```python
from build123d import *

# Parameters (mm, degrees)
SKETCH1_R           = 6.2
BOSS_EXTRUDE1_DEPTH = 5.4
SKETCH2_R           = 3
BOSS_EXTRUDE3_DEPTH = 102.1
BOSS_EXTRUDE4_START = 5.4
SKETCH4_R           = 6.2
BOSS_EXTRUDE4_DEPTH = 5.4
SKETCH5_R           = 6
BOSS_EXTRUDE5_DEPTH = 43.8


with BuildPart() as part:
    # Sketch1 → Boss-Extrude1 (new body)
    with BuildSketch(Plane.XY):
        with BuildLine():
            Line((0, 0), (-149.578947368, 0))
            ThreePointArc((-149.578947368, 0), (-174.878947368, -25.3), (-149.578947368, -50.6))
            Line((-149.578947368, -50.6), (130.421052632, -50.6))
            ThreePointArc((130.421052632, -50.6), (155.721052632, -25.3), (130.421052632, 0))
            Line((130.421052632, 0), (0, 0))
        make_face()
        with Locations(Location((130.421052632, -25.3, 0), (0, 0, 180))):
            Circle(SKETCH1_R, mode=Mode.SUBTRACT)
    extrude(amount=BOSS_EXTRUDE1_DEPTH)

    # Sketch2 → Boss-Extrude3 (add)
    with BuildSketch(Plane(origin=(0, 0, 0), x_dir=(-1, 0, 0), z_dir=(0, 0, -1))):
        with Locations(Location((-68.985809966, -25.3, 0), (0, 0, 180))):
            Circle(SKETCH2_R)
    extrude(amount=BOSS_EXTRUDE3_DEPTH)

    # Sketch4 → Boss-Extrude4 (add)
    with BuildSketch(Plane(origin=(0, 0, -102.1), x_dir=(-1, 0, 0), z_dir=(0, 0, -1)).offset(BOSS_EXTRUDE4_START)):
        with BuildLine():
            Line((-130.421052632, 0), (149.578947368, 0))
            ThreePointArc((149.578947368, 0), (174.878947368, -25.3), (149.578947368, -50.6))
            Line((149.578947368, -50.6), (-130.421052632, -50.6))
            ThreePointArc((-130.421052632, -50.6), (-155.721052632, -25.3), (-130.421052632, 0))
        make_face()
        with Locations((-130.421052632, -25.3)):
            Circle(SKETCH4_R, mode=Mode.SUBTRACT)
    extrude(amount=-BOSS_EXTRUDE4_DEPTH)

    # Sketch5 → Boss-Extrude5 (add)
    with BuildSketch(Plane.XY.offset(-102.1)):
        with Locations((-149.578947368, -25.3)):
            Circle(SKETCH5_R)
    boss_extrude5 = extrude(amount=BOSS_EXTRUDE5_DEPTH)

    # Mirror1: Boss-Extrude5 across plane
    add(boss_extrude5.mirror(Plane.XY.offset(-51.05)))


solid = part.part
```
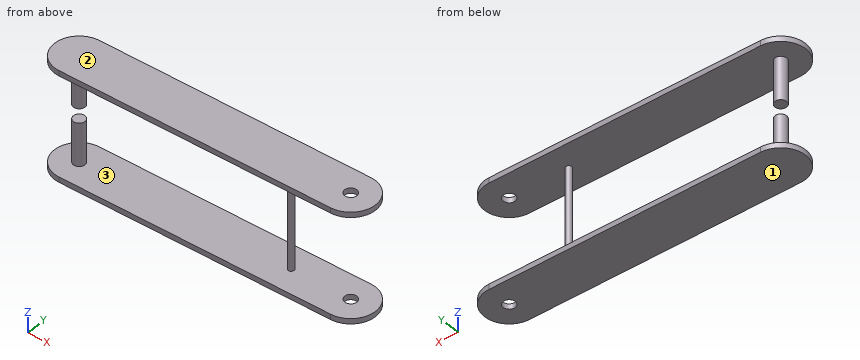
Source: CAD feature listing. Evaluate the final solid. Frame: model axes, mm. Face numbers are marked on the shaded views. Round coordinates to 2 decimals unless told otherwise and drop trailing zeros. Write each loop counter-clockwise with the first axis right and the second up, starting at its lowest first coordinate (ties: lowest second). Pieces come first, ordered by that corner, then holes. Notation, with made-up numbers: M 65.5,-20.75 L 94.5,-20.75 A26 ccw 94.5,8.25 Z; hole C 73.5,-19.75 d8. An arc over 180 degrees is marked long. Use CSV: the item, a comma, the result in double quotes. Start each with the question number.
Q1. Pull-direction query (Z, two-part tool) for the marked faces 1, 2 and 3; classes: +Z half, -Z half, draft (parallel to the pull), parting line (faces both ways), or undercut.
Q2. Cut plane C-C on y = -5. Output: boundary loops of the cut face in (x, z).
Q3. Cut plane B-B on y = -25.3. Output: boundary loops of the cut face in (x, z).
Q4. Line query: line 1 (Z direction, x = 122, y = -11); line 2 (X direction, y = -25, z = -104); line 3 (Y direction, x = -150, z = -77). Output: solid intervals per line, ascending. Write a range as from..to.
Q5. Cut plane A-A on x = -34.5. Output: boundary loops of the cut face in (y, z).
Q6. Cut plane D-D on z = -62. Output: boundary loops of the cut face in (x, y).
Results found:
1,face 1,"-Z half"
1,face 2,"+Z half"
1,face 3,"undercut"
2,outline,"M -164.68,-107.5 L 145.52,-107.5 L 145.52,-102.1 L -164.68,-102.1 Z; M -164.68,0 L 145.52,0 L 145.52,5.4 L -164.68,5.4 Z"
3,outline,"M -174.88,-107.5 L 124.22,-107.5 L 124.22,-102.1 L 71.99,-102.1 L 71.99,0 L 124.22,0 L 124.22,5.4 L -174.88,5.4 L -174.88,0 L -155.58,0 L -155.58,-43.8 L -143.58,-43.8 L -143.58,0 L 65.99,0 L 65.99,-102.1 L -143.58,-102.1 L -143.58,-58.3 L -155.58,-58.3 L -155.58,-102.1 L -174.88,-102.1 Z; M 136.62,-107.5 L 155.72,-107.5 L 155.72,-102.1 L 136.62,-102.1 Z; M 136.62,0 L 155.72,0 L 155.72,5.4 L 136.62,5.4 Z"
4,line 1,"-107.5..-102.1, 0..5.4"
4,line 2,"-174.88..124.23, 136.61..155.72"
4,line 3,"-31.29..-19.31"
5,outline,"M -50.6,-107.5 L 0,-107.5 L 0,-102.1 L -50.6,-102.1 Z; M -50.6,0 L 0,0 L 0,5.4 L -50.6,5.4 Z"
6,outline,"C -149.58,-25.3 d12; C 68.99,-25.3 d6"
